from build123d import *

# Parameters (mm, degrees)
SKETCH2_R           = 49.53
SKETCH2_R_2         = 48.26
BOSS_EXTRUDE1_DEPTH = 203.2
SKETCH4_W           = 95
SKETCH4_H           = 4
CUT_EXTRUDE1_DEPTH  = 4
CIRPATTERN1_COUNT   = 4


with BuildPart() as part:
    # Sketch2 → Boss-Extrude1 (new body)
    with BuildSketch(Plane(origin=(0, 0, 0), x_dir=(0, 0, -1), z_dir=(1, 0, 0))):
        Circle(SKETCH2_R)
        Circle(SKETCH2_R_2, mode=Mode.SUBTRACT)
    extrude(amount=BOSS_EXTRUDE1_DEPTH)

    # Sketch4 → Cut-Extrude1 (cut, symmetric)
    with BuildSketch(Plane.XY):
        with Locations((135.7, 47.53)):
            Rectangle(SKETCH4_W, SKETCH4_H)
    cut_extrude1 = extrude(amount=CUT_EXTRUDE1_DEPTH, both=True, mode=Mode.SUBTRACT)

    # CirPattern1: Cut-Extrude1 ×4 about axis
    cirpattern1_axis = Axis((0, 0, 0), (1, 0, 0))
    for i in range(1, CIRPATTERN1_COUNT):
        add(cut_extrude1.rotate(cirpattern1_axis, i * 360 / CIRPATTERN1_COUNT), mode=Mode.SUBTRACT)


solid = part.part
CAD build for the part. Positions are in the model's coordinates, mm. Round coordinates to 2 decimals unless told otherwise and drop trailing zeros. Write each loop counter-clockwise with the first axis right and the second up, starting at its lowest first coordinate (ties: lowest second). Pieces come first, ordered by that corner, then holes. Notation, with made-up numbers: M 66.25,85 L 95.25,85 A18 ccw 95.25,103 Z; hole C 38.5,6.25 d10. An arc over 180 degrees is marked long. Use a Markdown table: item, result. Add a question column.
1. Pull direction Y, two halves, no side cores. Call faces 1 (the face through (100.18, 14.5, -46.03)), 2 (the face through (100.18, 14.88, -47.24)), 3 (the face through (0, -47.5, -10.8)): released by +Y, released by -Y, zero draft, split by the parting line, or undercut.
2. Slice it at D-D on z = -13. Give the cut face in (x, y).
3. Flat gauge pins, fed straight in: P1, Ø4, axis at x = 55.5, y = 22.5, coming from the -Z side; P2, Ø12, axis at x = 175, y = 36, coming from the +Z side; P3, Ø3, axis at x = 38.5, y = 23.5, coming from the +Z side. Where does each tip first touch, or does it go through?
4. Slice it at A-A on z = 0. Give the cut face in (x, y), then the cut area to 3 significant figures.
5. Slice it at C-C on y = -32.5. Give the cut face in (x, z), then the cut area to 3 significant figures.
6. Slice it at B-B on x = 92.5. Give the cut face in (y, z).
7. Drill centre lines: probe 1 along Y at (x, z) = (62, 0); probe 2 along Y at (x, z) = (52, -1.5); probe 3 along Z at (x, y) = (103, -31.5). Where is each one in solid material? Low to high.
Reply:
| question | item | result |
|---|---|---|
| 1 | face 1 | undercut |
| 1 | face 2 | split by the parting line |
| 1 | face 3 | zero draft |
| 2 | outline | M 0,-47.79 L 203.2,-47.79 L 203.2,-46.48 L 0,-46.48 Z; M 0,46.48 L 203.2,46.48 L 203.2,47.79 L 0,47.79 Z |
| 3 | P1 | stops at z = -45.09 |
| 3 | P2 | stops at z = 39.41 |
| 3 | P3 | stops at z = 44.38 |
| 4 | outline | M 0,-49.53 L 88.2,-49.53 L 88.2,-48.26 L 0,-48.26 Z; M 0,48.26 L 88.2,48.26 L 88.2,49.53 L 0,49.53 Z; M 183.2,-49.53 L 203.2,-49.53 L 203.2,-48.26 L 183.2,-48.26 Z; M 183.2,48.26 L 203.2,48.26 L 203.2,49.53 L 183.2,49.53 Z |
| 4 | area | 275 mm^2 |
| 5 | outline | M 0,-37.38 L 203.2,-37.38 L 203.2,-35.68 L 0,-35.68 Z; M 0,35.68 L 203.2,35.68 L 203.2,37.38 L 0,37.38 Z |
| 5 | area | 691 mm^2 |
| 6 | outline | M -49.37,-4 A49.53 ccw -4,-49.37 L -4,-48.09 A48.26 cw -48.09,-4 Z; M -49.37,4 L -48.09,4 A48.26 cw -4,48.09 L -4,49.37 A49.53 ccw Z; M 4,-49.37 A49.53 ccw 49.37,-4 L 48.09,-4 A48.26 cw 4,-48.09 Z; M 4,48.09 A48.26 cw 48.09,4 L 49.37,4 A49.53 ccw 4,49.37 Z |
| 7 | probe 1 | y = -49.53 to -48.26, 48.26 to 49.53 |
| 7 | probe 2 | y = -49.51 to -48.24, 48.24 to 49.51 |
| 7 | probe 3 | z = -38.22 to -36.56, 36.56 to 38.22 |
